Geometry: final body of the model. Coordinates: model frame, mm. Face numbers are marked on the shaded views. A direction names the side the tool comes from. Round coordinates to 2 decimals unless told otherwise and drop trailing zeros. Write each loop counter-clockwise with the first axis right and the second up, starting at its lowest first coordinate (ties: lowest second). Pieces come first, ordered by that corner, then holes. Notation, with made-up numbers: (-27.75, 14.5) -> (-1.75, 14.5) arc R18 ccw to (-1.75, 43.5) -> close; hole circle Ø3 at (1.5, -3). An arc over 180 degrees is marked (long way). Use one line per item in the form item = value. Start each with the question number.
1. Cut plane C-C, the plane y = 0. Return the cut outline in (x, z) (3 decimals).
2. Reachability of the marked faces 1 and 2 from +Z, -Z, +X, -X, +Y, -Y: full face, straight path, thin tool, end or side. Return the list, or none.
3. Cut plane A-A, the plane x = 0. State how many separate pieces and enclosed holes the cut face has, plus the area to 3 significant figures.
4. Cut plane B-B, the plane z = 10. Return the cut outline in (x, y) (3 decimals).
5. Cut plane D-D, the plane z = 6. Return the cut outline in (x, y), plus the area to 3 significant figures.
6. Draft query along Y for the marked faces 3, 4 and 5. Return one class per face: pulls with the +Y half, pulls with the -Y half, needs draft (parallel to the pull), parting line crosses it, or undercut.
7. Pin query (flat end, axial travel): pin 1 Ø4 at (x, y) = (0, -12) entering from +Z; pin 2 Ø4.5 at (x, y) = (0.5, -1) entering from +Z; pin 3 Ø3 at (x, y) = (-7, 16) entering from +Z. Return the tip coordinate at first contact, or that it passes through.
8. Line query: L1, parallel to Y at x = 0, z = 0.5 (3 decimals); L2, parallel to Y at x = 0, z = 2.4 (3 decimals); L3, parallel to X at y = -8, z = 5.75. Output: solid intervals per line, ascending.
```python
from build123d import *

# Parameters (mm, degrees)
SKETCH1_W                        = 18
SKETCH1_H                        = 36
SKETCH1_R                        = 2.525
BOSS_EXTRUDE1_DEPTH              = 12
SHELL1_T                         = -3
SKETCH1_3_R                      = 2.525
CUT_EXTRUDE1_DEPTH               = 10
SKETCH2_R                        = 2.925
CUT_EXTRUDE2_DEPTH               = 1
FILLET1_R                        = 4
TAP_DRILL_FOR_M3_HELICOIL1_D     = 3.15
TAP_DRILL_FOR_M3_HELICOIL1_DEPTH = 3.3
TAP_DRILL_FOR_M3_HELICOIL1_TIP   = 0.946355475


with BuildPart() as part:
    # Sketch1 → Boss-Extrude1 (new body)
    # profile 1 of 4: a face of its own
    with BuildSketch(Plane.XY):
        Rectangle(SKETCH1_W, SKETCH1_H)
        with Locations((0, -12)):
            Circle(SKETCH1_R, mode=Mode.SUBTRACT)
        Circle(SKETCH1_R, mode=Mode.SUBTRACT)
        with Locations((0, 12)):
            Circle(SKETCH1_R, mode=Mode.SUBTRACT)
    # profile 2 of 4: a face of its own
    with BuildSketch(Plane.XY):
        with Locations((0, -12)):
            Circle(SKETCH1_R)
    # profile 3 of 4: a face of its own
    with BuildSketch(Plane.XY):
        Circle(SKETCH1_R)
    # profile 4 of 4: a face of its own
    with BuildSketch(Plane.XY):
        with Locations((0, 12)):
            Circle(SKETCH1_R)
    extrude(amount=BOSS_EXTRUDE1_DEPTH)

    # Shell1
    shell1_openings = [part.faces().sort_by_distance(p)[0] for p in [
        (0, 0, 12),
    ]]
    offset(amount=SHELL1_T, openings=shell1_openings, kind=Kind.INTERSECTION)

    # Sketch1_3 → Cut-Extrude1 (cut)
    with BuildSketch(Plane.XY):
        with Locations((0, 12)):
            Circle(SKETCH1_3_R)
        Circle(SKETCH1_3_R)
        with Locations((0, -12)):
            Circle(SKETCH1_3_R)
    extrude(amount=CUT_EXTRUDE1_DEPTH, mode=Mode.SUBTRACT)

    # Sketch2 → Cut-Extrude2 (cut)
    with BuildSketch(Plane.XY.offset(3)):
        with Locations((0, 12)):
            Circle(SKETCH2_R)
        Circle(SKETCH2_R)
        with Locations((0, -12)):
            Circle(SKETCH2_R)
    extrude(amount=-CUT_EXTRUDE2_DEPTH, mode=Mode.SUBTRACT)

    # Fillet1
    fillet1_edges = [part.edges().sort_by_distance(p)[0] for p in [
        (-6, -15, 7.5),
        (6, -15, 7.5),
        (6, 15, 7.5),
        (-6, 15, 7.5),
    ]]
    fillet(fillet1_edges, radius=FILLET1_R)

    # Tap Drill for M3 Helicoil1
    with Locations(Plane.XY.offset(12)):
        with Locations((7, -16), (-7, 16)):
            Hole(TAP_DRILL_FOR_M3_HELICOIL1_D / 2, depth=TAP_DRILL_FOR_M3_HELICOIL1_DEPTH)
            with Locations((0, 0, -(TAP_DRILL_FOR_M3_HELICOIL1_DEPTH + TAP_DRILL_FOR_M3_HELICOIL1_TIP / 2))):  # 118° drill point
                Cone(0, TAP_DRILL_FOR_M3_HELICOIL1_D / 2, TAP_DRILL_FOR_M3_HELICOIL1_TIP, mode=Mode.SUBTRACT)


solid = part.part
```
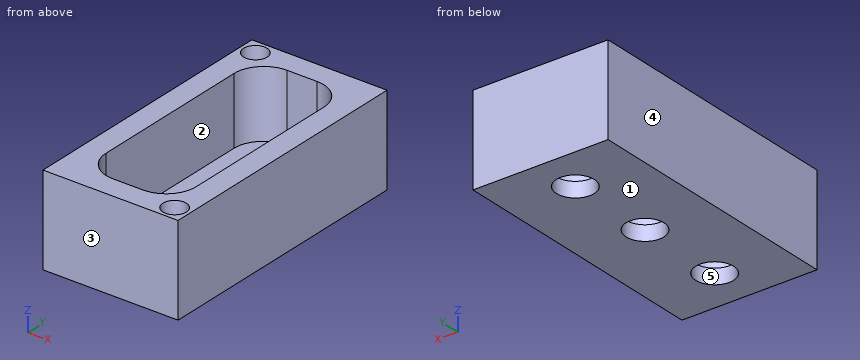
Outcome:
q1.outline = (-9, 0) -> (-2.525, 0) -> (-2.525, 2) -> (-2.925, 2) -> (-2.925, 3) -> (-6, 3) -> (-6, 12) -> (-9, 12) -> close; (2.525, 0) -> (9, 0) -> (9, 12) -> (6, 12) -> (6, 3) -> (2.925, 3) -> (2.925, 2) -> (2.525, 2) -> close
q2.face_1 = -Z, +X, -X, +Y, -Y
q2.face_2 = +Z
q3.separate_pieces = 4
q3.enclosed_holes = 0
q3.area = 114 mm^2
q4.outline = (-9, -18) -> (9, -18) -> (9, 18) -> (-9, 18) -> close; hole circle Ø3.15 at (-7, 16); hole (-6, -11) arc R4 ccw to (-2, -15) -> (2, -15) arc R4 ccw to (6, -11) -> (6, 11) arc R4 ccw to (2, 15) -> (-2, 15) arc R4 ccw to (-6, 11) -> close; hole circle Ø3.15 at (7, -16)
q5.outline = (-9, -18) -> (9, -18) -> (9, 18) -> (-9, 18) -> close; hole (-6, -11) arc R4 ccw to (-2, -15) -> (2, -15) arc R4 ccw to (6, -11) -> (6, 11) arc R4 ccw to (2, 15) -> (-2, 15) arc R4 ccw to (-6, 11) -> close
q5.area = 302 mm^2
q6.face_3 = pulls with the -Y half
q6.face_4 = needs draft
q6.face_5 = undercut
q7.pin_1 = through
q7.pin_2 = 3
q7.pin_3 = 8.65
q8.L1 = -18 to -14.525, -9.475 to -2.525, 2.525 to 9.475, 14.525 to 18
q8.L2 = -18 to -14.925, -9.075 to -2.925, 2.925 to 9.075, 14.925 to 18
q8.L3 = -9 to -6, 6 to 9
